The listing builds one solid part. Answer for the finished solid, in the listing's coordinates (mm). A direction names the side the tool comes from. Coordinates: 2 decimals unless noted, no trailing zeros. Order: outer loops, then holes, each group sorted by start corner. A loop starts at its lowest first (then second) coordinate and runs counter-clockwise, first axis right, second up. Notation, with made-up numbers: (58.25, 64.5) -> (96.25, 64.5) arc R16 cw to (96.25, 77.5) -> close; hole circle Ø5 at (84, -40). An arc over 180 degrees is marked (long way). One line per question, with ' | ' between items.
from build123d import *

# Parameters (mm, degrees)
SKETCH_W     = 47
SKETCH_H     = 41
PAD_DEPTH    = 1
SKETCH001_W  = 9
SKETCH001_H  = 15
PAD001_DEPTH = 11
SKETCH002_W  = 7
SKETCH002_H  = 6
PAD002_DEPTH = 9
SKETCH003_W  = 47
SKETCH003_H  = 41
PAD003_DEPTH = 4
SKETCH011_W  = 14
SKETCH011_H  = 7
PAD006_DEPTH = 6


with BuildPart() as part:
    # Sketch → Pad (new body)
    with BuildSketch(Plane.XY):
        Rectangle(SKETCH_W, SKETCH_H)
    extrude(amount=PAD_DEPTH)

    # Sketch001 (on Face6 of Pad) → Pad001 (join)
    with BuildSketch(Plane.XY.offset(1)):
        with Locations((9, -13)):
            Rectangle(SKETCH001_W, SKETCH001_H)
    extrude(amount=PAD001_DEPTH)

    # Sketch002 (on Face5 of Pad001) → Pad002 (join)
    with BuildSketch(Plane.XY.offset(1)):
        with Locations((-18.5, -17.5)):
            Rectangle(SKETCH002_W, SKETCH002_H)
    extrude(amount=PAD002_DEPTH)

    # Sketch003 (on Face5 of Pad002) → Pad003 (join)
    with BuildSketch(Plane.XY.offset(1)):
        Rectangle(SKETCH003_W, SKETCH003_H)
    extrude(amount=PAD003_DEPTH)

    # Sketch011 (on Face5 of Pad003) → Pad006 (join)
    with BuildSketch(Plane(origin=(0, 20.5, 0), x_dir=(-1, 0, 0), z_dir=(0, 1, 0))):
        with Locations((-4.5, 4.5)):
            Rectangle(SKETCH011_W, SKETCH011_H)
    extrude(amount=-PAD006_DEPTH)


solid = part.part
Item 1: Each of these flat-tipped pins is pushed along its axis until it touches: pin 1 Ø2 at (x, y) = (-2.5, 9) entering from +Z; pin 2 Ø6.5 at (x, y) = (-19, -18.5) entering from +Z; pin 3 Ø6.5 at (x, y) = (5, 16) entering from +Z. Where does it stop, or does it pass through?
Computed values:
pin 1: stops at z = 5 | pin 2: stops at z = 10 | pin 3: stops at z = 8
Item 2: Section B-B, the plane z = 9.25 is taken. Give the vertices of the cut face in (x, y).
Computed values:
outline: (-22, -20.5) -> (-15, -20.5) -> (-15, -14.5) -> (-22, -14.5) -> close; (4.5, -20.5) -> (13.5, -20.5) -> (13.5, -5.5) -> (4.5, -5.5) -> close
Item 3: Section D-D, the plane y = 16 is taken. Give the vertices of the cut face in (x, z).
Computed values:
outline: (-23.5, 0) -> (23.5, 0) -> (23.5, 5) -> (11.5, 5) -> (11.5, 8) -> (-2.5, 8) -> (-2.5, 5) -> (-23.5, 5) -> close
Item 4: Section A-A, the plane z = 5.75 is taken. Give the vertices of the cut face in (x, y).
Computed values:
outline: (-22, -20.5) -> (-15, -20.5) -> (-15, -14.5) -> (-22, -14.5) -> close; (-2.5, 14.5) -> (11.5, 14.5) -> (11.5, 20.5) -> (-2.5, 20.5) -> close; (4.5, -20.5) -> (13.5, -20.5) -> (13.5, -5.5) -> (4.5, -5.5) -> close
Item 5: Section C-C, the plane x = -21 is taken. Give the vertices of the cut face in (y, z).
Computed values:
outline: (-20.5, 0) -> (20.5, 0) -> (20.5, 5) -> (-14.5, 5) -> (-14.5, 10) -> (-20.5, 10) -> close
Item 6: For faces 4 (the face through (-22, -18, 7)), 5 (the face through (13.5, -13, 8)), 6 (the face through (11.5, 18, 6)), 7 (the face through (5, 18, 8)), 8 (the face through (-15, -18, 7)), determine the directions among +Z, -Z, +X, -X, +Y, -Y from which every point of the face is accessible in a straight line to the end or side of a thin tool.
Computed values:
face 4: +Z, -X, +Y, -Y | face 5: +Z, +X, +Y, -Y | face 6: +Z, +X, +Y | face 7: +Z, +X, -X, +Y | face 8: +Z, +Y, -Y
Item 7: Determine the mould class of faces 1 (the face through (5, 14.5, 7)), 2 (the face through (-19, -14.5, 7)), 3 (the face through (0, 0, 0)) for opening direction Y: pulls with the +Y half, pulls with the -Y half, needs draft (parallel to the pull), parting line crosses it, or undercut.
Computed values:
face 1: undercut | face 2: pulls with the +Y half | face 3: needs draft
Item 8: Find the intervals of material crossed by L1, parallel to X at y = -17, z = 5.25; L2, parallel to Z at x = -15.5, y = -3; L3, parallel to X at y = -11, z = 9.75, in increasing order.
Computed values:
L1: x = -22 to -15, 4.5 to 13.5 | L2: z = 0 to 5 | L3: x = 4.5 to 13.5
